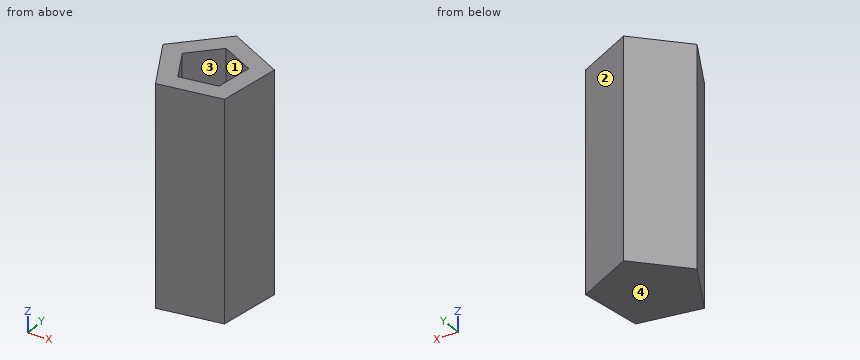
```python
from build123d import *

# Parameters (mm, degrees)
F1_DEPTH = 177.8
F2_T     = -14.1111111111


# Not quite as in the source:
# - a length typed as a fraction of an inch, garbled in the dataset ("3 / 203.2 mm" for 3/8 in), is restored


with BuildPart() as f1:
    # F0 (on Top) → F1 (new body)
    with BuildSketch(Plane.XY):
        Polygon((-6.8708224943, 42.663338416), (-42.6984469235, 6.6491561018), (-19.5182689713, -38.5539339486), (30.6354932977, -30.4767976821), (38.4520450914, 19.7182371128), align=None)
    extrude(amount=F1_DEPTH)

    # F2
    f2_openings = [f1.faces().sort_by_distance(p)[0] for p in [
        (0, 0, 177.8),
    ]]
    offset(amount=F2_T, openings=f2_openings)


solid = f1.part
```
Input: part model. Units: mm. Frame: model coordinates. Face numbers are marked on the shaded views. Coordinates: 2 decimals unless noted, no trailing zeros. Write each loop counter-clockwise with the first axis right and the second up, starting at its lowest first coordinate (ties: lowest second). Pieces come first, ordered by that corner, then holes.
1) Material intervals for line 1 along Y through (x, z) = (0.5, 25.5); line 2 along X through (y, z) = (6, 20.5); line 3 along Y through (x, z) = (16.5, 166), sorted ascending.
2) Section A-A on z = 156.5. Output: boundary loops of the cut face in (x, y).
3) Section B-B on x = 14. Output: boundary loops of the cut face in (y, z).
4) Mould query, pull axis Y, two halves, no side actions, for the marked faces 1, 2, 3 and 4. Classes: pulls with the +Y half, pulls with the -Y half, needs draft (parallel to the pull), parting line crosses it, or undercut.
5) Pin query (flat end, axial travel): pin 1 Ø4 at (y, z) = (-26, 26) entering from +X; pin 2 Ø6 at (y, z) = (-10, 110) entering from -X; pin 3 Ø4 at (y, z) = (-23, 108) entering from +X. Return the tip coordinate at first contact, or that it passes through.
6) Section D-D on x = 32.5. Output: boundary loops of the cut face in (y, z), and give its area (3 significant figures).
7) Section C-C on y = -7. Output: boundary loops of the cut face in (x, z), and give its area (3 significant figures).
Check result:
1. line 1: y = -35.33 to -21.04, 23.12 to 38.93
1. line 2: x = -42.37 to -23.44, 22.03 to 36.32
1. line 3: y = -32.75 to -18.46, 15.02 to 30.83
2. outline: (-42.7, 6.65) - (-19.52, -38.55) - (30.64, -30.48) - (38.45, 19.72) - (-6.87, 42.66) - close; hole (-25.46, 3.97) - (-11.64, -22.99) - (18.27, -18.18) - (22.93, 11.76) - (-4.1, 25.44) - close
3. outline: (-33.16, 0) - (32.1, 0) - (32.1, 177.8) - (16.28, 177.8) - (16.28, 14.11) - (-18.86, 14.11) - (-18.86, 177.8) - (-33.16, 177.8) - close
4. face 1: undercut
4. face 2: pulls with the +Y half
4. face 3: undercut
4. face 4: needs draft
5. pin 1: stops at x = 31.64
5. pin 2: stops at x = -35.7
5. pin 3: stops at x = 32.11
6. outline: (-18.5, 0) - (22.73, 0) - (22.73, 177.8) - (-18.5, 177.8) - close
6. area: 7,330 mm2
7. outline: (-35.7, 0) - (34.29, 0) - (34.29, 177.8) - (20.01, 177.8) - (20.01, 14.11) - (-19.84, 14.11) - (-19.84, 177.8) - (-35.7, 177.8) - close
7. area: 5,920 mm2
